```python
from build123d import *

# Parameters (mm, degrees)
SKETCH1_W           = 387.4
SKETCH1_H           = 169.4
BOSS_EXTRUDE1_DEPTH = 2.5
SKETCH3_W           = 40
SKETCH3_H           = 2.8
CUT_EXTRUDE2_DEPTH  = 2
CUT_EXTRUDE3_DEPTH  = 10
CUT_EXTRUDE4_DEPTH  = 3.5
CHAMFER1_SIZE       = 1
CHAMFER2_SIZE       = 1
CUT_EXTRUDE5_DEPTH  = 2


with BuildPart() as part:
    # Sketch1 → Boss-Extrude1 (new body)
    with BuildSketch(Plane(origin=(0, 0, 0), x_dir=(1, 0, 0), z_dir=(0, 1, 0))):
        Rectangle(SKETCH1_W, SKETCH1_H)
    extrude(amount=BOSS_EXTRUDE1_DEPTH)

    # Sketch3 → Cut-Extrude2 (cut)
    with BuildSketch(Plane(origin=(0, 2.5, 0), x_dir=(1, 0, 0), z_dir=(0, 1, 0))):
        with Locations((137.5, 80.1)):
            Rectangle(SKETCH3_W, SKETCH3_H)
        Polygon((-157.5, 81), (-157.5, 78.7), (-117.5, 78.2), (-117.5, 81), align=None)
    extrude(amount=-CUT_EXTRUDE2_DEPTH, mode=Mode.SUBTRACT)

    # Sketch4 → Cut-Extrude3 (cut)
    with BuildSketch(Plane.XZ):
        Polygon((31.499996994, 73.5), (105.5, 30.5), (182.7, 30.5), (182.7, -73.7), (-182.7, -73.7), (-182.7, 30.5), (-105.5, 30.5), (-31.499996994, 73.5), align=None)
    extrude(amount=-CUT_EXTRUDE3_DEPTH, mode=Mode.SUBTRACT)

    # Sketch7 → Cut-Extrude4 (cut, through all)
    with BuildSketch(Plane.XZ):
        Polygon((193.7, 41.5), (105.5, 41.5), (31.499996994, 84.5), (-31.499996994, 84.5), (-105.5, 41.5), (-193.7, 41.5), (-193.7, 84.7), (193.7, 84.7), align=None)
    extrude(amount=-CUT_EXTRUDE4_DEPTH, mode=Mode.SUBTRACT)

    # Chamfer1
    chamfer1_edges = [part.edges().sort_by_distance(p)[0] for p in [
        (-193.7, 0, -21.6),
        (0, 0, -84.7),
        (193.7, 0, -21.6),
        (-149.6, 0, 41.5),
        (-68.499998497, 0, 63),
        (0, 0, 84.5),
        (68.499998497, 0, 63),
        (149.6, 0, 41.5),
    ]]
    chamfer(chamfer1_edges, length=CHAMFER1_SIZE)

    # Chamfer2
    chamfer2_edges = [part.edges().sort_by_distance(p)[0] for p in [
        (0, 0, 73.5),
        (-68.499998497, 0, 52),
        (-144.1, 0, 30.5),
        (-182.7, 0, -21.6),
        (0, 0, -73.7),
        (182.7, 0, -21.6),
        (144.1, 0, 30.5),
        (68.499998497, 0, 52),
    ]]
    chamfer(chamfer2_edges, length=CHAMFER2_SIZE)

    # Sketch9 → Cut-Extrude5 (cut)
    with BuildSketch(Plane(origin=(0, 2.5, 0), x_dir=(1, 0, 0), z_dir=(0, 1, 0))):
        Polygon((-70.007252094, -59.593875696), (-52.714747454, -69.642222987), (-51.20749536, -67.048347291), (-85.79250464, -46.951652709), (-87.299756734, -49.545528405), align=None)
        Polygon((70.007252094, -59.593875696), (52.714747454, -69.642222987), (51.20749536, -67.048347291), (85.79250464, -46.951652709), (87.299756734, -49.545528405), align=None)
    extrude(amount=-CUT_EXTRUDE5_DEPTH, mode=Mode.SUBTRACT)


solid = part.part
```
Part model, mm, in its own coordinate system. A direction names the side the tool comes from. Round coordinates to 2 decimals unless told otherwise and drop trailing zeros. Loops run counter-clockwise (first coordinate to the right, second up) from the corner with the lowest first, then second, coordinate; pieces in that order, holes last.
1. Flat gauge pins, fed straight in: pin 1 (0.6 mm diameter, centred on x = -145, y = 2, fed in from +Z); pin 2 (0.8 mm diameter, centred on x = -136, z = -79, fed in from +Y). Where does each tip first touch, or does it go through?
Solutions:
pin 1: stops at z = 41.5
pin 2: stops at y = 0.5
2. Drill centre lines: line 1 along X through (y, z) = (0.6, 50.5); line 2 along Z through (x, y) = (111, 1.9); line 3 along Z through (x, y) = (-54.5, 1.4). Where is each one in solid material? Low to high.
Solutions:
line 1: x = -89.22 to -85.66, -79.69 to -71.88, 71.88 to 79.69, 85.66 to 89.22
line 2: z = -84.7 to -73.7, 30.5 to 41.5
line 3: z = -84.7 to -73.7, 60.14 to 65.14, 68.6 to 71.14
3. Two-plate mould, pull along X, no slides. Class faces 1 (the face through (68.888, 0.507, 62.204)), 2 (the face through (-67.85, 0.51, 62.81)), 3 (the face through (13, 0, -75)), 4 (the face through (69.77, 1.51, 59.73)): pulls with the +X half, pulls with the -X half, needs draft (parallel to the pull), parting line crosses it, or undercut.
Solutions:
face 1: pulls with the +X half
face 2: pulls with the -X half
face 3: needs draft
face 4: undercut
4. Slice it at B-B (y = 2.05). Count the separate pieces of the cut face and the enclosed holes in it, and give its area (3 significant figures).
Solutions:
separate pieces: 1
enclosed holes: 5
area: 10,400 mm2
5. Slice it at D-D (x = 8). Give the cut face in (y, z), and give its area (3 significant figures).
Solutions:
outline: (0, -83.7) - (1, -84.7) - (2.5, -84.7) - (2.5, -73.7) - (1, -73.7) - (0, -74.7) - close; (0, 74.5) - (1, 73.5) - (2.5, 73.5) - (2.5, 84.5) - (1, 84.5) - (0, 83.5) - close
area: 53.0 mm2
6. Slice it at C-C (x = 136.5). Give the cut face in (y, z).
Solutions:
outline: (0, -83.7) - (1, -84.7) - (2.5, -84.7) - (2.5, -81.5) - (0.5, -81.5) - (0.5, -78.7) - (2.5, -78.7) - (2.5, -73.7) - (1, -73.7) - (0, -74.7) - close; (0, 31.5) - (1, 30.5) - (2.5, 30.5) - (2.5, 41.5) - (1, 41.5) - (0, 40.5) - close
7. 3-axis set-ups, long thin cutter, end or side, ignore diameter. For faces 5 (the face through (-69.02, 1.74, 51.7)), 6 (the face through (68.26, 1.51, 57.14)), 7 (the face through (-69.15, 0.51, 52.19)): which of +Z, -Z, +X, -X, +Y, -Y reach the whole face in a straight line?
Solutions:
face 5: +Y, -Y
face 6: +Y
face 7: -Y
8. Slice it at A-A (z = -31). Give the cut face in (x, y).
Solutions:
outline: (-193.7, 1) - (-192.7, 0) - (-183.7, 0) - (-182.7, 1) - (-182.7, 2.5) - (-193.7, 2.5) - close; (182.7, 1) - (183.7, 0) - (192.7, 0) - (193.7, 1) - (193.7, 2.5) - (182.7, 2.5) - close
